from build123d import *

# Parameters (mm, degrees)
F0_R     = 20
F0_R_2   = 1.5
F1_DEPTH = 5
F4_R     = 14.613565
F5_DEPTH = 5


with BuildPart() as f1:
    # F0 (on Top) → F1 (new body)
    with BuildSketch(Plane.XY):
        Circle(F0_R)
        Circle(F0_R_2, mode=Mode.SUBTRACT)
    extrude(amount=F1_DEPTH)

    # F2 (on Front) → F3 (revolve, intersect)
    with BuildSketch(Plane.XZ):
        Polygon((20, 0.538248), (20, 4.461752), (19.430714, 5), (18.09014, 5), (7.885276, 0), (19.430714, 0), align=None)
    revolve(axis=Axis((0, 0, 2.5), (0, 0, 1)), mode=Mode.INTERSECT)

    # F4 (on Top) → F5 (join, through all)
    with BuildSketch(Plane.XY):
        with Locations((0, -2.476576)):
            Circle(F4_R)
    extrude(amount=F5_DEPTH)


solid = f1.part
Verification items for the finished model (mm, model axes). Coordinates: 2 decimals unless noted, no trailing zeros. Order: outer loops, then holes, each group sorted by start corner. A loop starts at its lowest first (then second) coordinate and runs counter-clockwise, first axis right, second up.
1. Release check for a two-part mould opening along Y. For faces 1 (the face through (-4.336, -19.524, 2.527)), 2 (the face through (-1.618, 12.32, 2.225)), 3 (the face through (13, -13, 5)) record: +Y half, -Y half, draft (parallel to the pull), parting line (faces both ways), or undercut.
Results found:
face 1: parting line
face 2: undercut
face 3: draft
2. Sectioned sample at B-B, the plane y = 0. Record the cut outline in (x, z).
Results found:
outline: (-20, 0.54) - (-19.43, 0) - (19.43, 0) - (20, 0.54) - (20, 4.46) - (19.43, 5) - (18.09, 5) - (14.4, 3.19) - (14.4, 5) - (-14.4, 5) - (-14.4, 3.19) - (-18.09, 5) - (-19.43, 5) - (-20, 4.46) - close
3. Scan lines: line 1 (Y direction, x = -6, z = 3.4); line 2 (X direction, y = 6, z = 2.6); line 3 (Y direction, x = -14, z = 1.1). Record each from-to range of solid material in increasing order.
Results found:
line 1: y = -19.08 to 10.85, 13.56 to 19.08
line 2: x = -19.08 to 19.08
line 3: y = -14.28 to 14.28
4. Sectioned sample at A-A, the plane x = 0. Record the cut outline in (y, z).
Results found:
outline: (-20, 0.54) - (-19.43, 0) - (19.43, 0) - (20, 0.54) - (20, 4.46) - (19.43, 5) - (18.09, 5) - (12.14, 2.08) - (12.14, 5) - (-17.09, 5) - (-17.09, 4.51) - (-18.09, 5) - (-19.43, 5) - (-20, 4.46) - close
5. Go/stop test with flat-tipped pins: pin 1 Ø1 at (x, z) = (14.5, 3.5) entering from +Y; pin 2 Ø1.5 at (x, z) = (9, 4.5) entering from +Y; pin 3 Ø1 at (x, y) = (-11, 9) entering from +Z. Record where each tip stops, or that it passes through.
Results found:
pin 1: stops at y = 14.28
pin 2: stops at y = 18.22
pin 3: stops at z = 3.35
